Design review of the part built by this model. Coordinates are the model's own, in mm. Give positions to 0.01 mm unless a question says otherwise; leave off trailing zeros. Use CSV: the item, a comma, the result in double quotes.
from build123d import *

# Parameters (mm, degrees)
SKIZZE1_W                       = 206
SKIZZE1_H                       = 236
AUFSATZ_LINEAR_AUSTRAGEN1_DEPTH = 3
SCHNITT_LINEAR_AUSTRAGEN2_DEPTH = 3
SKIZZE3_R                       = 1.65
SCHNITT_LINEAR_AUSTRAGEN3_DEPTH = 3


with BuildPart() as part:
    # Skizze1 → Aufsatz-Linear austragen1 (new body)
    with BuildSketch(Plane(origin=(0, 0, 0), x_dir=(1, 0, 0), z_dir=(0, 1, 0))):
        Rectangle(SKIZZE1_W, SKIZZE1_H)
    extrude(amount=AUFSATZ_LINEAR_AUSTRAGEN1_DEPTH)

    # Skizze2 → Schnitt-Linear austragen2 (cut)
    with BuildSketch(Plane(origin=(0, 3, 0), x_dir=(1, 0, 0), z_dir=(0, 1, 0))):
        with BuildLine():
            ThreePointArc((-21.427553093, 91.819125025), (-40.305086528, 79.305086528), (-52.819125025, 60.427553093))
            Line((-52.819125025, 60.427553093), (-21.427553093, 91.819125025))
        make_face()
        with BuildLine():
            ThreePointArc((-55.866928677, 50.30868163), (-56.534459002, 46.27014067), (-56.910435609, 42.194106886))
            Line((-56.910435609, 42.194106886), (-3.194106886, 95.910435609))
            ThreePointArc((-3.194106886, 95.910435609), (-7.27014067, 95.534459002), (-11.30868163, 94.866928677))
            Line((-11.30868163, 94.866928677), (-55.866928677, 50.30868163))
        make_face()
        with BuildLine():
            ThreePointArc((-56.870693274, 35.162781409), (-56.569218878, 32.005468167), (-56.092595564, 28.869811308))
            Line((-56.092595564, 28.869811308), (10.130188692, 95.092595564))
            ThreePointArc((10.130188692, 95.092595564), (6.994531833, 95.569218878), (3.837218591, 95.870693274))
            Line((3.837218591, 95.870693274), (-56.870693274, 35.162781409))
        make_face()
        with BuildLine():
            ThreePointArc((-54.749577763, 23.141761296), (-53.910125432, 20.487885699), (-52.942116187, 17.878155061))
            Line((-52.942116187, 17.878155061), (21.121844939, 91.942116187))
            ThreePointArc((21.121844939, 91.942116187), (18.512114301, 92.910125432), (15.858238704, 93.749577763))
            Line((15.858238704, 93.749577763), (-54.749577763, 23.141761296))
        make_face()
        with BuildLine():
            ThreePointArc((-50.733032764, 13.016170672), (-49.499198499, 10.736430728), (-48.162990305, 8.515145319))
            Line((-48.162990305, 8.515145319), (30.484854681, 87.162990305))
            ThreePointArc((30.484854681, 87.162990305), (28.263569272, 88.499198499), (25.983829328, 89.733032764))
            Line((25.983829328, 89.733032764), (-50.733032764, 13.016170672))
        make_face()
        with BuildLine():
            ThreePointArc((-45.258164778, 4.348903034), (-43.688596063, 2.389802322), (-42.034290815, 0.501709185))
            Line((-42.034290815, 0.501709185), (38.498290815, 81.034290815))
            ThreePointArc((38.498290815, 81.034290815), (36.610197678, 82.688596063), (34.651096966, 84.258164778))
            Line((34.651096966, 84.258164778), (-45.258164778, 4.348903034))
        make_face()
        with BuildLine():
            Line((42.034290815, 77.498290815), (-38.498290815, -3.034290815))
            ThreePointArc((-38.498290815, -3.034290815), (-36.610197678, -4.688596063), (-34.651096966, -6.258164778))
            Line((-34.651096966, -6.258164778), (45.258164778, 73.651096966))
            ThreePointArc((45.258164778, 73.651096966), (43.688596063, 75.610197678), (42.034290815, 77.498290815))
        make_face()
        with BuildLine():
            Line((48.162990305, 69.484854681), (-30.484854681, -9.162990305))
            ThreePointArc((-30.484854681, -9.162990305), (-28.263569272, -10.499198499), (-25.983829328, -11.733032764))
            Line((-25.983829328, -11.733032764), (50.733032764, 64.983829328))
            ThreePointArc((50.733032764, 64.983829328), (49.499198499, 67.263569272), (48.162990305, 69.484854681))
        make_face()
        with BuildLine():
            Line((52.942116187, 60.121844939), (-21.121844939, -13.942116187))
            ThreePointArc((-21.121844939, -13.942116187), (-18.512114301, -14.910125432), (-15.858238704, -15.749577763))
            Line((-15.858238704, -15.749577763), (54.749577763, 54.858238704))
            ThreePointArc((54.749577763, 54.858238704), (53.910125432, 57.512114301), (52.942116187, 60.121844939))
        make_face()
        with BuildLine():
            Line((56.092595564, 49.130188692), (-10.130188692, -17.092595564))
            ThreePointArc((-10.130188692, -17.092595564), (-6.994531833, -17.569218878), (-3.837218591, -17.870693274))
            Line((-3.837218591, -17.870693274), (56.870693274, 42.837218591))
            ThreePointArc((56.870693274, 42.837218591), (56.569218878, 45.994531833), (56.092595564, 49.130188692))
        make_face()
        with BuildLine():
            Line((56.910435609, 35.805893114), (3.194106886, -17.910435609))
            ThreePointArc((3.194106886, -17.910435609), (7.27014067, -17.534459002), (11.30868163, -16.866928677))
            Line((11.30868163, -16.866928677), (55.866928677, 27.69131837))
            ThreePointArc((55.866928677, 27.69131837), (56.534459002, 31.72985933), (56.910435609, 35.805893114))
        make_face()
        with BuildLine():
            Line((52.819125025, 17.572446907), (21.427553093, -13.819125025))
            ThreePointArc((21.427553093, -13.819125025), (40.305086528, -1.305086528), (52.819125025, 17.572446907))
        make_face()
    extrude(amount=-SCHNITT_LINEAR_AUSTRAGEN2_DEPTH, mode=Mode.SUBTRACT)

    # Skizze3 → Schnitt-Linear austragen3 (cut)
    with BuildSketch(Plane(origin=(0, 3, 0), x_dir=(1, 0, 0), z_dir=(0, 1, 0))):
        with Locations((-100.7, 115.7)):
            Circle(SKIZZE3_R)
        with Locations((100.7, 115.7)):
            Circle(SKIZZE3_R)
        with Locations((100.7, -115.7)):
            Circle(SKIZZE3_R)
        with Locations((-100.7, -115.7)):
            Circle(SKIZZE3_R)
    extrude(amount=-SCHNITT_LINEAR_AUSTRAGEN3_DEPTH, mode=Mode.SUBTRACT)


solid = part.part
(1) We need section A-A on y = 1.9. Count the separate pieces of the cut face and the enclosed holes in it, then the cut area to 3 significant figures.
A:
separate pieces,"1"
enclosed holes,"16"
area,"43,500 mm²"
(2) Wall thickness on line 1 along Z through (x, y) = (-100.7, 0.7); line 2 along X through (y, z) = (0.9, 115.7); line 3 along X through (y, z) = (1.65, -87): over which ranges is each line inside the solid? List them lowest first. Write a range as [from, to].
A:
line 1,"[-118, -117.35], [-114.05, 114.05], [117.35, 118]"
line 2,"[-103, -102.35], [-99.05, 99.05], [102.35, 103]"
line 3,"[-103, -30.74], [-26.25, -19.18], [-12.1, -5.03], [2.04, 9.11], [16.18, 23.25], [30.32, 103]"
(3) The part is to be moulded in two halves that separate along Z. For faces 1 (the flat face through (-1, 3, 25)), 2 (the cylindrical face through (-40.08, 1.52, -79.53)), 3 (the flat face through (-18.95, 1.52, -58.94)), say which applies: released by +Z, released by -Z, zero draft, split by the parting line, or undercut.
A:
face 1,"zero draft"
face 2,"undercut"
face 3,"undercut"
